Verification items for the finished model (mm, model axes). A direction names the side the tool comes from. Give positions to 0.01 mm unless a question says otherwise; leave off trailing zeros. Write each loop counter-clockwise with the first axis right and the second up, starting at its lowest first coordinate (ties: lowest second). Pieces come first, ordered by that corner, then holes. Notation, with made-up numbers: (83, 67) -> (95, 67) arc R29 cw to (95, 94) -> close; hole circle Ø6 at (-34, -22). An arc over 180 degrees is marked (long way). Use CSV: the item, a comma, the result in double quotes. Start each with the question number.
```python
from build123d import *

# Parameters (mm, degrees)
SKETCH006_W          = 44.958
SKETCH006_H          = 67.818
PAD003_DEPTH         = 3.81
SKETCH007_W          = 41.1226
SKETCH007_H          = 63.881
PAD004_DEPTH         = 0.762
SKETCH008_R          = 4.022821
SKETCH008_R_2        = 1.5875
SKETCH008_R_3        = 3.643361
PAD005_DEPTH         = 17.018
PAD006_DEPTH         = 6.35
SKETCH010_R          = 1.5875
POCKET003_DEPTH      = 17.019
POCKET003_DEPTH_BACK = 3.811
SKETCH011_R          = 3.556
POCKET004_DEPTH      = 2.54


with BuildPart() as part:
    # Sketch006 (on DatumPlane) → Pad003 (new body)
    with BuildSketch(Plane.XY.offset(18.829)):
        with Locations((20.32, 31.75)):
            Rectangle(SKETCH006_W, SKETCH006_H)
    extrude(amount=PAD003_DEPTH)

    # Sketch007 (on DatumPlane) → Pad004 (join)
    with BuildSketch(Plane.XY.offset(18.829)):
        with Locations((20.3835, 31.7627)):
            Rectangle(SKETCH007_W, SKETCH007_H)
    extrude(amount=-PAD004_DEPTH)

    # Sketch008 (on DatumPlane) → Pad005 (join)
    with BuildSketch(Plane.XY.offset(18.829)):
        with Locations((3.819621, 59.680379)):
            Circle(SKETCH008_R)
        with Locations((3.819621, 59.680379)):
            Circle(SKETCH008_R_2, mode=Mode.SUBTRACT)
        with Locations((37.301439, 48.057955)):
            Circle(SKETCH008_R_3)
        with Locations((37.301439, 48.057955)):
            Circle(SKETCH008_R_2, mode=Mode.SUBTRACT)
    extrude(amount=-PAD005_DEPTH)

    # Sketch009 (on DatumPlane) → Pad006 (join)
    with BuildSketch(Plane.XY.offset(18.829)):
        Polygon((0, 63.5), (0, 19.05), (40.9448, 19.05), (40.9448, 63.7032), align=None)
    extrude(amount=-PAD006_DEPTH)

    # Sketch010 (on DatumPlane) → Pocket003 (cut, two sides)
    with BuildSketch(Plane.XY.offset(18.829)) as pocket003_sk:
        with Locations((3.819621, 59.680379)):
            Circle(SKETCH010_R)
        with Locations((37.301439, 48.057955)):
            Circle(SKETCH010_R)
    extrude(amount=-POCKET003_DEPTH, mode=Mode.SUBTRACT)
    extrude(pocket003_sk.sketch, amount=POCKET003_DEPTH_BACK, mode=Mode.SUBTRACT)

    # Sketch011 (on Face5 of Pocket003) → Pocket004 (cut)
    with BuildSketch(Plane.XY.offset(22.639)):
        with Locations((3.819621, 59.680379)):
            Circle(SKETCH011_R)
        with Locations((37.301439, 48.057955)):
            Circle(SKETCH011_R)
    extrude(amount=-POCKET004_DEPTH, mode=Mode.SUBTRACT)


solid = part.part
```
(1) Section check D-D on z = 14.5. Give the number of separate pieces and of enclosed holes in the cut face, then the cut area to 3 significant figures.
(2) Thickness scan on line 1 (Z direction, x = 25, y = 34); line 2 (X direction, y = 35, z = 14.25); line 3 (Y direction, x = 38, z = 6.25). Record the ranges inside material, lowest first. Write a range as from..to.
(3) Go/stop test with flat-tipped pins: pin 1 (4 mm diameter, centred on x = 32, y = 9.5, fed in from -Z); pin 2 (2 mm diameter, centred on x = 2.5, y = 59.5, fed in from +Z); pin 3 (12.5 mm diameter, centred on x = 25.5, y = 41, fed in from -Z). Record where each tip stops, or that it passes through.
(4) Section check B-B on x = 23.5. Record the cut outline in (y, z).
(5) Draft check along Y on faces 1 (the face through (22, 10, 18.067)), 2 (the face through (3.48, 58.13, 10.83)), 3 (the face through (39.26, 51.13, 7.22)). Enter one of: released by +Y, released by -Y, zero draft, split by the parting line, or undercut.
(6) Section check A-A on z = 8. Record the cut outline in (x, y) (1 decimal).
(7) Set-up check for faces 4 (the face through (42.799, 31, 21)), 5 (the face through (0, 62, 15)), 6 (the face through (20, 19.05, 15)), 7 (the face through (39, 47, 20.099)), 8 (the face through (40.945, 38, 16)): record each of +Z, -Z, +X, -X, +Y, -Y from which the full face is reachable in a straight line by a thin tool's end or side.
(8) Section check C-C on y = 54.5. Record the cut outline in (x, z), then the cut area to 3 significant figures.
Data:
1,separate pieces,"1"
1,enclosed holes,"2"
1,area,"1,810 mm2"
2,line 1,"z = 12.48..22.64"
2,line 2,"x = 0..40.94"
2,line 3,"y = 44.48..46.63, 49.48..51.63"
3,pin 1,"stops at z = 18.07"
3,pin 2,"stops at z = 20.1"
3,pin 3,"stops at z = 12.48"
4,outline,"(-2.16, 18.83) -> (-0.18, 18.83) -> (-0.18, 18.07) -> (19.05, 18.07) -> (19.05, 12.48) -> (63.62, 12.48) -> (63.62, 18.07) -> (63.7, 18.07) -> (63.7, 18.83) -> (65.66, 18.83) -> (65.66, 22.64) -> (-2.16, 22.64) -> close"
5,face 1,"zero draft"
5,face 2,"undercut"
5,face 3,"split by the parting line"
6,outline,"circle Ø8 at (3.8, 59.7); circle Ø7.3 at (37.3, 48.1); hole circle Ø3.2 at (3.8, 59.7); hole circle Ø3.2 at (37.3, 48.1)"
7,face 4,"+Z, -Z, +X, +Y, -Y"
7,face 5,"-Z, -X, +Y"
7,face 6,"-Z, +X, -X, -Y"
7,face 7,"+Z"
7,face 8,"-Z, +X, +Y, -Y"
8,outline,"(-2.16, 18.83) -> (-0.18, 18.83) -> (-0.18, 18.07) -> (0, 18.07) -> (0, 12.48) -> (40.94, 12.48) -> (40.94, 18.83) -> (42.8, 18.83) -> (42.8, 22.64) -> (-2.16, 22.64) -> close"
8,area,"431 mm2"
